Input: part model. Units: mm. Frame: model coordinates. Coordinates: 2 decimals unless noted, no trailing zeros. Order: outer loops, then holes, each group sorted by start corner. A loop starts at its lowest first (then second) coordinate and runs counter-clockwise, first axis right, second up. Notation, with made-up numbers: (-28, 22) -> (-3, 22) arc R23 cw to (-3, 38) -> close; hole circle Ø3 at (40.5, -10). An arc over 180 degrees is marked (long way). Use CSV: the item, a comma, the result in double quotes. Start each with the question number.
```python
from build123d import *

# Parameters (mm, degrees)
SKETCH_W      = 40
SKETCH_H      = 10
PAD_DEPTH     = 10
SKETCH001_R   = 0.85
HOLE_DEPTH    = 25
SKETCH002_R   = 0.9
HOLE001_DEPTH = 25
SKETCH003_R   = 0.95
HOLE002_DEPTH = 25
SKETCH004_R   = 1
HOLE003_DEPTH = 25
SKETCH005_R   = 1.05
HOLE004_DEPTH = 25
SKETCH006_R   = 1.1
HOLE005_DEPTH = 25
SKETCH007_R   = 1.15
HOLE006_DEPTH = 25
SKETCH008_R   = 1.2
HOLE007_DEPTH = 25
SKETCH009_R   = 1.25
HOLE008_DEPTH = 25
SKETCH010_R   = 1.2
HOLE009_DEPTH = 25
SKETCH011_R   = 1.5
HOLE010_DEPTH = 25


with BuildPart() as part:
    # Sketch → Pad (new body)
    with BuildSketch(Plane.XY):
        Rectangle(SKETCH_W, SKETCH_H)
    extrude(amount=PAD_DEPTH)

    # Sketch001 (on Face6 of Pad) → Hole (cut)
    with BuildSketch(Plane.XY.offset(10)):
        with Locations((-18.51713, 0)):
            Circle(SKETCH001_R)
    extrude(amount=-HOLE_DEPTH, mode=Mode.SUBTRACT)

    # Sketch002 (on Face6 of Pad) → Hole001 (cut)
    with BuildSketch(Plane.XY.offset(10)):
        with Locations((-15.935542, 0)):
            Circle(SKETCH002_R)
    extrude(amount=-HOLE001_DEPTH, mode=Mode.SUBTRACT)

    # Sketch003 (on Face6 of Pad) → Hole002 (cut)
    with BuildSketch(Plane.XY.offset(10)):
        with Locations((-13.345876, 0)):
            Circle(SKETCH003_R)
    extrude(amount=-HOLE002_DEPTH, mode=Mode.SUBTRACT)

    # Sketch004 (on Face6 of Pad) → Hole003 (cut)
    with BuildSketch(Plane.XY.offset(10)):
        with Locations((-10.761359, 0)):
            Circle(SKETCH004_R)
    extrude(amount=-HOLE003_DEPTH, mode=Mode.SUBTRACT)

    # Sketch005 (on Face6 of Pad) → Hole004 (cut)
    with BuildSketch(Plane.XY.offset(10)):
        with Locations((-7.973536, 0)):
            Circle(SKETCH005_R)
    extrude(amount=-HOLE004_DEPTH, mode=Mode.SUBTRACT)

    # Sketch006 (on Face6 of Pad) → Hole005 (cut)
    with BuildSketch(Plane.XY.offset(10)):
        with Locations((-5.038025, 0)):
            Circle(SKETCH006_R)
    extrude(amount=-HOLE005_DEPTH, mode=Mode.SUBTRACT)

    # Sketch007 (on Face6 of Pad) → Hole006 (cut)
    with BuildSketch(Plane.XY.offset(10)):
        with Locations((-1.486799, 0)):
            Circle(SKETCH007_R)
    extrude(amount=-HOLE006_DEPTH, mode=Mode.SUBTRACT)

    # Sketch008 (on Face6 of Pad) → Hole007 (cut)
    with BuildSketch(Plane.XY.offset(10)):
        with Locations((1.512776, 0)):
            Circle(SKETCH008_R)
    extrude(amount=-HOLE007_DEPTH, mode=Mode.SUBTRACT)

    # Sketch009 (on Face6 of Pad) → Hole008 (cut)
    with BuildSketch(Plane.XY.offset(10)):
        with Locations((4.793622, 0)):
            Circle(SKETCH009_R)
    extrude(amount=-HOLE008_DEPTH, mode=Mode.SUBTRACT)

    # Sketch010 (on Face6 of Pad) → Hole009 (cut)
    with BuildSketch(Plane.XY.offset(10)):
        with Locations((15.717695, 0)):
            Circle(SKETCH010_R)
    extrude(amount=-HOLE009_DEPTH, mode=Mode.SUBTRACT)

    # Sketch011 (on Face5 of Hole009) → Hole010 (cut)
    with BuildSketch(Plane.XY.offset(10)):
        with Locations((10.428464, 0)):
            Circle(SKETCH011_R)
    extrude(amount=-HOLE010_DEPTH, mode=Mode.SUBTRACT)


solid = part.part
```
1. Section B-B on z = 8. State how many separate pieces and enclosed holes the cut face has, then the cut area to 3 significant figures.
2. Pull-direction query (Y, two-part tool) for faces 1 (the face through (-6.137, 0.048, 5.07)), 2 (the face through (-6.972, 0.315, 5.07)), 3 (the face through (-20, 0, 5)), 4 (the face through (0, 5, 5)); classes: released by +Y, released by -Y, zero draft, split by the parting line, or undercut.
3. Material intervals for line 1 along Y through (x, z) = (-8.5, 6); line 2 along Y through (x, z) = (-5, 3.25), sorted ascending.
4. Contact query for a flat-ended pin moving along its axis: P1, Ø4, axis at x = 1.51, y = 0, coming from the +Z side. Output: stop coordinate, or through.
5. Section A-A on x = 1. Return loops of the section in (y, z).
6. Section D-D on x = 11. Return loops of the section in (y, z), then the cut area to 3 significant figures.
Values follow:
1,separate pieces,"1"
1,enclosed holes,"11"
1,area,"357 mm2"
2,face 1,"undercut"
2,face 2,"undercut"
2,face 3,"zero draft"
2,face 4,"released by +Y"
3,line 1,"y = -5 to -0.91, 0.91 to 5"
3,line 2,"y = -5 to -1.1, 1.1 to 5"
4,P1,"stops at z = 10"
5,outline,"(-5, 0) -> (-1.08, 0) -> (-1.08, 10) -> (-5, 10) -> close; (1.08, 0) -> (5, 0) -> (5, 10) -> (1.08, 10) -> close"
6,outline,"(-5, 0) -> (-1.39, 0) -> (-1.39, 10) -> (-5, 10) -> close; (1.39, 0) -> (5, 0) -> (5, 10) -> (1.39, 10) -> close"
6,area,"72.3 mm2"
